Work out the finished part from the listing and answer in its coordinate system (mm). A direction names the side the tool comes from. Round coordinates to 2 decimals unless told otherwise and drop trailing zeros. Write each loop counter-clockwise with the first axis right and the second up, starting at its lowest first coordinate (ties: lowest second). Pieces come first, ordered by that corner, then holes. Notation, with made-up numbers: (52, 6.5) -> (111, 6.5) arc R27 cw to (111, 39.5) -> close; hole circle Ø9 at (13, 40.5). An arc over 180 degrees is marked (long way). Answer as a JSON object with one key per item and string values. Group by question number.
from build123d import *

# Parameters (mm, degrees)
SKETCH_1_R               = 5
SKETCH_1_R_2             = 3.1
EXTRUDE_1_DEPTH          = 20
SKETCH_2_W               = 45
SKETCH_2_H               = 4
EXTRUDE_2_DEPTH          = 3.5
SKETCH_4_R               = 1.6
CUT_EXTRUDE_2_DEPTH      = 14
FILLET_1_R               = 3
SKETCH_5_R               = 1.6
CUT_EXTRUDE_3_DEPTH      = 6
CUT_EXTRUDE_3_DEPTH_BACK = 6
SKETCH_3_R               = 3.1
CUT_EXTRUDE_4_DEPTH      = 8.0000001
CUT_EXTRUDE_4_DEPTH_BACK = 14.0000001


with BuildPart() as part:
    # 草图1 → 凸台-拉伸1 (new body)
    with BuildSketch(Plane(origin=(0, 0, 0), x_dir=(1, 0, 0), z_dir=(0, 1, 0))):
        Circle(SKETCH_1_R)
        Circle(SKETCH_1_R_2, mode=Mode.SUBTRACT)
    extrude(amount=EXTRUDE_1_DEPTH)

    # 草图2 → 凸台-拉伸2 (add, symmetric)
    with BuildSketch(Plane.XY):
        with Locations((0, 11)):
            Rectangle(SKETCH_2_W, SKETCH_2_H)
    extrude(amount=EXTRUDE_2_DEPTH, both=True)

    # 草图4 → 切除-拉伸2 (cut, through all)
    with BuildSketch(Plane(origin=(0, 13, 0), x_dir=(1, 0, 0), z_dir=(0, 1, 0))):
        with Locations((-18, 0)):
            Circle(SKETCH_4_R)
        with Locations((18, 0)):
            Circle(SKETCH_4_R)
    extrude(amount=-CUT_EXTRUDE_2_DEPTH, mode=Mode.SUBTRACT)

    # 圆角1
    fillet_1_edges = [part.edges().sort_by_distance(p)[0] for p in [
        (22.5, 11, 3.5),
        (-22.5, 11, 3.5),
        (-22.5, 11, -3.5),
        (22.5, 11, -3.5),
    ]]
    fillet(fillet_1_edges, radius=FILLET_1_R)

    # 草图5 → 切除-拉伸3 (cut, two sides)
    with BuildSketch(Plane.XY) as cut_extrude_3_sk:
        with Locations((0, 15)):
            Circle(SKETCH_5_R)
    extrude(amount=CUT_EXTRUDE_3_DEPTH, mode=Mode.SUBTRACT)
    extrude(cut_extrude_3_sk.sketch, amount=-CUT_EXTRUDE_3_DEPTH_BACK, mode=Mode.SUBTRACT)

    # 草图3 → 切除-拉伸4 (cut, two sides)
    with BuildSketch(Plane(origin=(0, 13, 0), x_dir=(1, 0, 0), z_dir=(0, 1, 0))) as cut_extrude_4_sk:
        Circle(SKETCH_3_R)
    extrude(amount=CUT_EXTRUDE_4_DEPTH, mode=Mode.SUBTRACT)
    extrude(cut_extrude_4_sk.sketch, amount=-CUT_EXTRUDE_4_DEPTH_BACK, mode=Mode.SUBTRACT)


solid = part.part
1) For a pull along Y with two mould halves and no side action, classify faces 4 (the face through (1.526, 15.481, 3.814)), 5 (the face through (-12, 11, 3.5)), 6 (the face through (-0.1, 0, 3.3)) as released by +Y, released by -Y, zero draft, split by the parting line, or undercut.
2) A cutting plane is placed at B-B on y = 15. Determine the outline of the cut face in (x, z), plus the area to 3 significant figures.
3) A cutting plane is placed at A-A on z = 0. Determine the outline of the cut face in (x, y).
4) A tool of negligible diameter and unlimited length cuts with its end or side. For faces 1 (the face through (21.6, 11.03, -2.64)), 2 (the face through (-12, 11, -3.5)), 3 (the face through (2.307, 9.86, 4.436)), from which of +Z, -Z, +X, -X, +Y, -Y can it reach the whole face along a straight path? Write none if from no direction.
5) Each of these flat-tipped pins is pushed along its axis until it touches: P1, Ø2, axis at x = -17, z = -0.5, coming from the -Y side; P2, Ø5.5, axis at x = 17.5, z = 1.5, coming from the +Y side; P3, Ø3, axis at x = -18, z = 0, coming from the +Y side; P4, Ø2, axis at x = 14.5, y = 10.5, coming from the -Z side. Where does it stop, or does it pass through?
6) A cutting plane is placed at D-D on x = 18. Determine the outline of the cut face in (y, z).
7) Straight lines are drawn through the part: L1, parallel to Y at x = 0, z = 4.15; L2, parallel to X at y = 10.75, z = 0; L3, parallel to X at y = 9.75, z = -0.5. For each, find the intervals that lie inside material, in ascending order.
8) A cutting plane is placed at C-C on x = 0. Determine the outline of the cut face in (y, z).
Established:
{
 "1": {"face 4": "undercut", "face 5": "zero draft", "face 6": "released by -Y"},
 "2": {"outline": "(-1.6, -4.74) -> (-1.6, -2.66) arc R3.1 cw to (-1.6, 2.66) -> (-1.6, 4.74) arc R5 ccw to start; (1.6, -4.74) arc R5 ccw to (1.6, 4.74) -> (1.6, 2.66) arc R3.1 cw to (1.6, -2.66) -> close", "area": "35.8 mm²"},
 "3": {"outline": "(-22.5, 9) -> (-19.6, 9) -> (-19.6, 13) -> (-22.5, 13) -> close; (-16.4, 9) -> (-5, 9) -> (-5, 0) -> (-3.1, 0) -> (-3.1, 20) -> (-5, 20) -> (-5, 13) -> (-16.4, 13) -> close; (3.1, 0) -> (5, 0) -> (5, 9) -> (16.4, 9) -> (16.4, 13) -> (5, 13) -> (5, 20) -> (3.1, 20) -> close; (19.6, 9) -> (22.5, 9) -> (22.5, 13) -> (19.6, 13) -> close"},
 "4": {"face 1": "-Z, +X, +Y, -Y", "face 2": "-Z, -X, +Y, -Y", "face 3": "none"},
 "5": {"P1": "stops at y = 9", "P2": "stops at y = 13", "P3": "passes through", "P4": "stops at z = -3.5"},
 "6": {"outline": "(9, -3.5) -> (13, -3.5) -> (13, -1.6) -> (9, -1.6) -> close; (9, 1.6) -> (13, 1.6) -> (13, 3.5) -> (9, 3.5) -> close"},
 "7": {"L1": "y = 0 to 13.4, 16.6 to 20", "L2": "x = -22.5 to -19.6, -16.4 to -3.1, 3.1 to 16.4, 19.6 to 22.5", "L3": "x = -22.5 to -19.52, -16.48 to -3.06, 3.06 to 16.48, 19.52 to 22.5"},
 "8": {"outline": "(0, -5) -> (13.4, -5) -> (13.4, -3.1) -> (0, -3.1) -> close; (0, 3.1) -> (13.4, 3.1) -> (13.4, 5) -> (0, 5) -> close; (16.6, -5) -> (20, -5) -> (20, -3.1) -> (16.6, -3.1) -> close; (16.6, 3.1) -> (20, 3.1) -> (20, 5) -> (16.6, 5) -> close"}
}
